The model under review builds one solid part; all positions refer to its coordinate system, in mm. Face numbers are marked on the shaded views. Give positions to 0.01 mm unless a question says otherwise; leave off trailing zeros. Loops run counter-clockwise (first coordinate to the right, second up) from the corner with the lowest first, then second, coordinate; pieces in that order, holes last. Notation, with made-up numbers: (10.25, -4.75) - (63.25, -4.75) arc R22 ccw to (63.25, 14.25) - close; hole circle Ø4 at (36.5, 30.25). An arc over 180 degrees is marked (long way). Answer as a JSON object with one key per item and string values.
from build123d import *

# Parameters (mm, degrees)
SKETCH2_W           = 302.006
SKETCH2_H           = 136.906
BOSS_EXTRUDE1_DEPTH = 12.7
SKETCH3_W           = 317.5
SKETCH3_H           = 152.4
BOSS_EXTRUDE2_DEPTH = 12.7
SKETCH4_W           = 289.306
SKETCH4_H           = 124.206
CUT_EXTRUDE1_DEPTH  = 12.7
CUT_EXTRUDE3_REACH  = 311.626
FILLET1_R           = 12.7


with BuildPart() as part:
    # Sketch2 → Boss-Extrude1 (new body)
    with BuildSketch(Plane.XY):
        Rectangle(SKETCH2_W, SKETCH2_H)
    extrude(amount=BOSS_EXTRUDE1_DEPTH)

    # Sketch3 → Boss-Extrude2 (add)
    with BuildSketch(Plane(origin=(0, 0, 0), x_dir=(-1, 0, 0), z_dir=(0, 0, -1))):
        with Locations((0.127, -0.127)):
            Rectangle(SKETCH3_W, SKETCH3_H)
    extrude(amount=BOSS_EXTRUDE2_DEPTH)

    # Sketch4 → Cut-Extrude1 (cut)
    with BuildSketch(Plane.XY.offset(12.7)):
        Rectangle(SKETCH4_W, SKETCH4_H)
    extrude(amount=-CUT_EXTRUDE1_DEPTH, mode=Mode.SUBTRACT)

    # Sketch5 → Cut-Extrude3 (cut, up to next)
    with BuildSketch(Plane.ZY.offset(151.003), mode=Mode.PRIVATE) as cut_extrude3_sk1:
        with BuildLine():
            Line((12.7, -45.72), (0, -45.72))
            Line((0, -45.72), (0, -38.608))
            Line((0, -38.608), (12.7, -38.608))
            ThreePointArc((12.7, -38.608), (16.256, -42.164), (12.7, -45.72))
        make_face()
    cut_extrude3_tool1 = extrude(cut_extrude3_sk1.sketch, amount=-CUT_EXTRUDE3_REACH, mode=Mode.PRIVATE) & part.part
    add(cut_extrude3_tool1.solids().sort_by_distance((-151.003, -42.164, 7.766768))[0], mode=Mode.SUBTRACT)

    # Fillet1
    fillet1_edges = [part.edges().sort_by_distance(p)[0] for p in [
        (-158.877, -76.327, -6.35),
        (-158.877, 76.073, -6.35),
        (158.623, 76.073, -6.35),
        (158.623, -76.327, -6.35),
        (-144.653, 62.103, 6.35),
        (144.653, 62.103, 6.35),
        (144.653, -62.103, 6.35),
        (-144.653, -62.103, 6.35),
        (-151.003, 68.453, 6.35),
        (151.003, 68.453, 6.35),
        (151.003, -68.453, 6.35),
        (-151.003, -68.453, 6.35),
    ]]
    fillet(fillet1_edges, radius=FILLET1_R)


solid = part.part
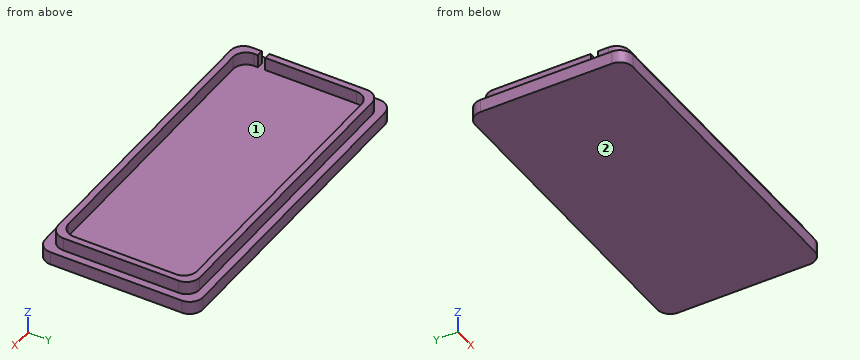
Q1. The part is to be moulded in two halves that separate along Y. For the marked faces 1 and 2, say which applies: +Y half, -Y half, draft (parallel to the pull), parting line (faces both ways), or undercut.
Results:
{"face 1": "undercut", "face 2": "draft"}
Q2. Consider section A-A, the plane x = 15.5. State the section outline as (y, z) points.
Results:
{"outline": "(-76.33, -12.7) - (76.07, -12.7) - (76.07, 0) - (68.45, 0) - (68.45, 12.7) - (62.1, 12.7) - (62.1, 0) - (-62.1, 0) - (-62.1, 12.7) - (-68.45, 12.7) - (-68.45, 0) - (-76.33, 0) - close"}
Q3. Consider section B-B, the plane y = 27. State the section outline as (x, z) points.
Results:
{"outline": "(-158.88, -12.7) - (158.62, -12.7) - (158.62, 0) - (151, 0) - (151, 12.7) - (144.65, 12.7) - (144.65, 0) - (-144.65, 0) - (-144.65, 12.7) - (-151, 12.7) - (-151, 0) - (-158.88, 0) - close"}
Q4. Consider section C-C, the plane z = 7. State the section outline as (x, y) points, plus the area to 3 significant figures.
Results:
{"outline": "(-151, -55.75) arc R12.7 ccw to (-138.3, -68.45) - (138.3, -68.45) arc R12.7 ccw to (151, -55.75) - (151, 55.75) arc R12.7 ccw to (138.3, 68.45) - (-138.3, 68.45) arc R12.7 ccw to (-151, 55.75) - (-151, -38.61) - (-144.65, -38.61) - (-144.65, 49.4) arc R12.7 cw to (-131.95, 62.1) - (131.95, 62.1) arc R12.7 cw to (144.65, 49.4) - (144.65, -49.4) arc R12.7 cw to (131.95, -62.1) - (-131.95, -62.1) arc R12.7 cw to (-144.65, -49.4) - (-144.65, -45.72) - (-151, -45.72) - close", "area": "5,370 mm^2"}
Q5. To check wall thickness, follow probe 1 along Y at (x, z) = (103, 6.5); probe 2 along X at (y, z) = (-3, 3.5); probe 3 along X at (y, z) = (-45, 10.75). State the ranges of each line that lie inside material, in increasing order. Write a range as [from, to].
Results:
{"probe 1": "y = [-68.45, -62.1], [62.1, 68.45]", "probe 2": "x = [-151, -144.65], [144.65, 151]", "probe 3": "x = [144.65, 151]"}
Q6. Clearance check with flat-ended pins moving along their axes: pin 1 Ø5 at (x, z) = (-148, 4) entering from -Y; pin 2 Ø6.5 at (x, z) = (-56, 7.5) entering from +Y; pin 3 Ø4 at (x, y) = (-29, -23) entering from +Z. State where each tip first meets the part, or that it passes through.
Results:
{"pin 1": "stops at y = -66.22", "pin 2": "stops at y = 68.45", "pin 3": "stops at z = 0"}
